Verification items for the finished model (mm, model axes). Face numbers are marked on the shaded views. A direction names the side the tool comes from. Coordinates: 2 decimals unless noted, no trailing zeros. Write each loop counter-clockwise with the first axis right and the second up, starting at its lowest first coordinate (ties: lowest second). Pieces come first, ordered by that corner, then holes. Notation, with made-up numbers: (81.25, 86.25) -> (107.25, 86.25) arc R8 cw to (107.25, 98.25) -> close; hole circle Ø11 at (-8, -35). An arc over 180 degrees is marked (long way). Answer in a Markdown table with one row per item.
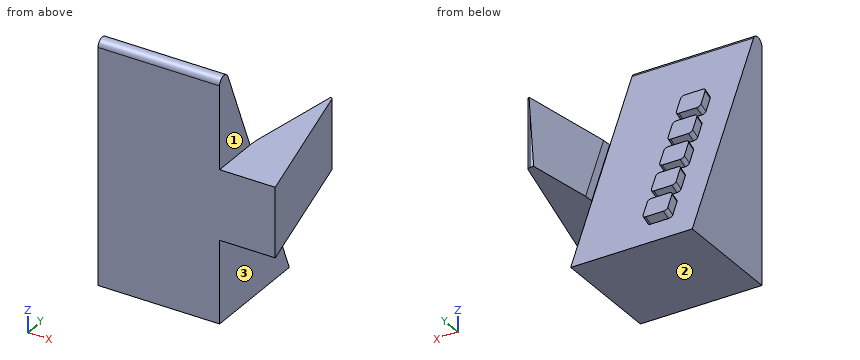
```python
from build123d import *

# Parameters (mm, degrees)
BOSS_EXTRUDE1_DEPTH = 88.9
SKETCH3_W           = 18.049999968
SKETCH3_H           = 18.049999968
BOSS_EXTRUDE2_DEPTH = 6.35
FILLET1_R           = 2.54
FILLET2_R           = 5.08
BOSS_EXTRUDE3_DEPTH = 40.64
CAVITY1_START       = 93.019234599
CAVITY1_DEPTH       = 75.946275307
CUT_EXTRUDE1_DEPTH  = 181.905623168
FILLET3_R           = 2.54


# Read off the part's stored shape, not the designer's step: Cavity1
with BuildPart() as part:
    # Sketch2 → Boss-Extrude1 (new body)
    with BuildSketch(Plane(origin=(0, 0, 0), x_dir=(0, 0, -1), z_dir=(1, 0, 0))):
        Polygon((0, 0), (196.85, 81.537939753), (196.85, 0), align=None)
    extrude(amount=-BOSS_EXTRUDE1_DEPTH)

    # Sketch3 → Boss-Extrude2 (add)
    with BuildSketch(Plane(origin=(0, 0, 0), x_dir=(1, 0, 0), z_dir=(0, 0.9238795325112891, 0.3826834323650843))):
        with Locations((-60.317000016, 184.485904644)):
            Rectangle(SKETCH3_W, SKETCH3_H)
        with Locations((-60.317000016, 159.085904644)):
            Rectangle(SKETCH3_W, SKETCH3_H)
        with Locations((-60.317000016, 133.685904644)):
            Rectangle(SKETCH3_W, SKETCH3_H)
        with Locations((-60.317000016, 108.285904644)):
            Rectangle(SKETCH3_W, SKETCH3_H)
        with Locations((-60.317000016, 82.885904644)):
            Rectangle(SKETCH3_W, SKETCH3_H)
    extrude(amount=BOSS_EXTRUDE2_DEPTH)

    # Fillet1
    fillet1_edges = [part.edges().sort_by_distance(p)[0] for p in [
        (-69.342, 76.986734699, -177.565744205),
        (-69.342, 70.079298757, -160.889718673),
        (-51.292000032, 70.079298757, -160.889718673),
        (-51.292000032, 76.986734699, -177.565744205),
        (-51.292000032, 67.266575517, -154.09920408),
        (-69.342, 67.266575517, -154.09920408),
        (-69.342, 60.359139575, -137.423178547),
        (-51.292000032, 60.359139575, -137.423178547),
        (-51.292000032, 57.546416335, -130.632663954),
        (-69.342, 57.546416335, -130.632663954),
        (-69.342, 50.638980393, -113.956638422),
        (-51.292000032, 50.638980393, -113.956638422),
        (-51.292000032, 47.826257152, -107.166123828),
        (-69.342, 47.826257152, -107.166123828),
        (-69.342, 40.918821211, -90.490098296),
        (-51.292000032, 40.918821211, -90.490098296),
        (-51.292000032, 38.10609797, -83.699583702),
        (-69.342, 38.10609797, -83.699583702),
        (-69.342, 31.198662028, -67.02355817),
        (-51.292000032, 31.198662028, -67.02355817),
    ]]
    fillet(fillet1_edges, radius=FILLET1_R)

    # Fillet2
    fillet2_edges = [part.edges().sort_by_distance(p)[0] for p in [
        (-44.45, 0, 0),
    ]]
    fillet(fillet2_edges, radius=FILLET2_R)

    # Sketch4 → Boss-Extrude3 (add)
    with BuildSketch(Plane(origin=(0, 0, 0), x_dir=(0, 0, -1), z_dir=(1, 0, 0))):
        Polygon((111.19444231, 0), (85.79444231, 0), (85.79444231, 111.76), (136.59444231, 111.76), (136.59444231, 0), align=None)
    extrude(amount=BOSS_EXTRUDE3_DEPTH)

    # Cavity1 outline → Cavity1 (cut)
    with BuildSketch(Plane(origin=(0, 0, 0), x_dir=(1, 0, 0), z_dir=(0, 0.38268343236508323, -0.9238795325112895)).offset(CAVITY1_START)):
        Polygon((0.339752359, -6.447958985), (0, -0.376615902), (0, -72), (11.89834583, -72), (11.619866439, -70.420664892), align=None)
    extrude(amount=CAVITY1_DEPTH, mode=Mode.SUBTRACT)

    # Sketch8 → Cut-Extrude1 (cut, through all)
    with BuildSketch(Plane.XY.offset(-85.79444231)):
        Polygon((12.889866439, 111.76), (40.64, 0), (40.64, 111.76), align=None)
    extrude(amount=-CUT_EXTRUDE1_DEPTH, mode=Mode.SUBTRACT)

    # Fillet3
    fillet3_edges = [part.edges().sort_by_distance(p)[0] for p in [
        (12.889866439, 111.76, -111.19444231),
    ]]
    fillet(fillet3_edges, radius=FILLET3_R)


solid = part.part
```
1. Sectioned sample at C-C, the plane z = -74.5. Record the cut outline in (x, y), and give its area (3 significant figures).
Findings below:
| item | result |
|---|---|
| outline | (-88.9, 0) -> (0, 0) -> (0, 30.86) -> (-51.29, 30.86) -> (-51.29, 37.73) -> (-69.34, 37.73) -> (-69.34, 30.86) -> (-88.9, 30.86) -> close |
| area | 2,870 mm² |
2. Go/stop test with flat-tipped pins: pin 1 (5 mm diameter, centred on x = -24.5, z = -120, fed in from +Y); pin 2 (1 mm diameter, centred on y = 79.5, z = -123.5, fed in from -X); pin 3 (3 mm diameter, centred on y = 52.5, z = -119, fed in from -X). Record where each tip stops, or that it passes through.
Findings below:
| item | result |
|---|---|
| pin 1 | stops at y = 50.74 |
| pin 2 | stops at x = 3.73 |
| pin 3 | stops at x = -69.34 |
3. Sectioned sample at D-D, the plane x = -77. Record the cut outline in (y, z), and give its area (3 significant figures).
Findings below:
| item | result |
|---|---|
| outline | (0, -196.85) -> (81.54, -196.85) -> (9.77, -23.59) arc R5.08 ccw to (0, -25.54) -> close |
| area | 7,930 mm² |
4. Material ranges on probe 1 along X at (y, z) = (23, -155); probe 2 along Z at (x, y) = (8, 65.5); probe 3 along Z at (x, y) = (-39.5, 57.5), recorded low to high. Write a range as from..to.
Findings below:
| item | result |
|---|---|
| probe 1 | x = -88.9..0 |
| probe 2 | z = -136.59..-85.79 |
| probe 3 | z = -196.85..-138.82 |
5. Access from +Z, -Z, +X, -X, +Y, -Y to the whole of each face (thin tool, end or side, straight path). Record for the marked faces 1, 2 and 3.
Findings below:
| item | result |
|---|---|
| face 1 | +Z, +X, +Y, -Y |
| face 2 | -Z, +X, -X, +Y, -Y |
| face 3 | -Z, +X, +Y, -Y |
6. Sectioned sample at B-B, the plane y = 18.5. Record the cut outline in (x, z).
Findings below:
| item | result |
|---|---|
| outline | (-88.9, -196.85) -> (0, -196.85) -> (0, -136.59) -> (36.05, -136.59) -> (36.05, -85.79) -> (0, -85.79) -> (0, -44.66) -> (-88.9, -44.66) -> close |
7. Sectioned sample at A-A, the plane x = -60.5. Record the cut outline in (y, z), and give its area (3 significant figures).
Findings below:
| item | result |
|---|---|
| outline | (0, -196.85) -> (81.54, -196.85) -> (74.05, -178.78) -> (79.92, -176.35) -> (73.01, -159.67) -> (67.15, -162.1) -> (64.33, -155.31) -> (70.2, -152.88) -> (63.29, -136.21) -> (57.43, -138.64) -> (54.61, -131.85) -> (60.48, -129.42) -> (53.57, -112.74) -> (47.71, -115.17) -> (44.89, -108.38) -> (50.76, -105.95) -> (43.85, -89.28) -> (37.99, -91.71) -> (35.17, -84.91) -> (41.04, -82.48) -> (34.13, -65.81) -> (28.27, -68.24) -> (9.77, -23.59) arc R5.08 ccw to (0, -25.54) -> close |
| area | 8,500 mm² |
